```python
from build123d import *

# Parameters (mm, degrees)
F3_DEPTH = 1.3


with BuildPart() as f1:
    # F0 (on Front) → F1 (revolve)
    with BuildSketch(Plane.XZ):
        Polygon((-2.75, 0), (-1.5, 0), (-1.5, -10), (0, -10), (0, 0), (0, 3), (-2.75, 3), align=None)
    revolve(axis=Axis((0, 0, -5), (0, 0, 1)))

    # F2 (on face) → F3 (cut)
    with BuildSketch(Plane.XY.offset(3)):
        Polygon((-1.25, 0.721688), (-1.25, -0.721688), (0, -1.443376), (1.25, -0.721688), (1.25, 0.721688), (0, 1.443376), align=None)
    extrude(amount=-F3_DEPTH, mode=Mode.SUBTRACT)


solid = f1.part
```
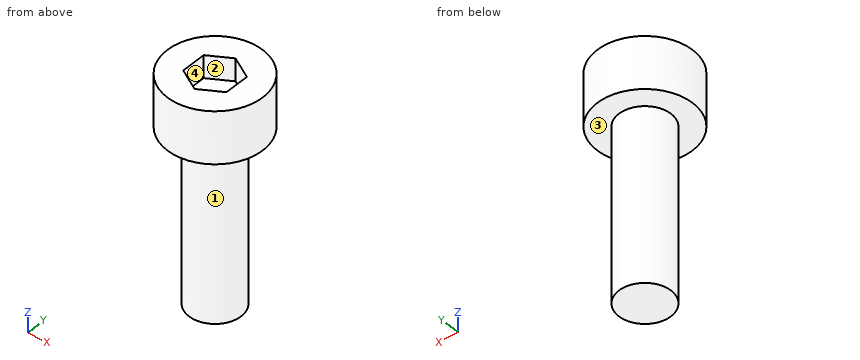
For this review, take the finished solid that the model builds, in its own axes (mm). Face numbers are marked on the shaded views. Give positions to 0.01 mm unless a question says otherwise; leave off trailing zeros. Write each loop counter-clockwise with the first axis right and the second up, starting at its lowest first coordinate (ties: lowest second). Pieces come first, ordered by that corner, then holes.
Item 1: Insertion check: P1, Ø0.6, axis at y = 0.5, z = 2, coming from the +X side; P2, Ø1, axis at x = 0, y = 0.5, coming from the +Z side; P3, Ø1.5, axis at x = 1.5, y = -2, coming from the -Z side. Each pin has a flat end and moves straight along its axis. Give the tip position at first contact, or say it passes through.
Item 2: Wall thickness on probe 1 along Z at (x, y) = (1.95, 1.5); probe 2 along Z at (x, y) = (-1.15, 0.4); probe 3 along Y at (x, z) = (0.55, 2.75): over which ranges is each line inside the solid? List them lowest first.
Item 3: Take a section at A-A (y = 0). Give the boundary of the cut face in (x, z).
Item 4: The part is to be moulded in two halves that separate along Y. For the marked faces 1, 2, 3 and 4, say which applies: +Y half, -Y half, draft (parallel to the pull), parting line (faces both ways), or undercut.
Item 5: Take a section at C-C (z = 1.25). Give the boundary of the cut face in (x, y).
Item 6: Take a section at D-D (y = -2.1). Give the boundary of the cut face in (x, z).
Item 7: Take a section at B-B (x = -0.6). Give the boundary of the cut face in (y, z).
Established:
1. P1: stops at x = 2.74
1. P2: stops at z = 1.7
1. P3: stops at z = 0
2. probe 1: z = 0 to 3
2. probe 2: z = -10 to 1.7
2. probe 3: y = -2.69 to -1.13, 1.13 to 2.69
3. outline: (-2.75, 0) - (-1.5, 0) - (-1.5, -10) - (1.5, -10) - (1.5, 0) - (2.75, 0) - (2.75, 3) - (1.25, 3) - (1.25, 1.7) - (-1.25, 1.7) - (-1.25, 3) - (-2.75, 3) - close
4. face 1: parting line
4. face 2: undercut
4. face 3: draft
4. face 4: undercut
5. outline: circle Ø5.5 at (0, 0)
6. outline: (-1.78, 0) - (1.78, 0) - (1.78, 3) - (-1.78, 3) - close
7. outline: (-2.68, 0) - (-1.37, 0) - (-1.37, -10) - (1.37, -10) - (1.37, 0) - (2.68, 0) - (2.68, 3) - (1.1, 3) - (1.1, 1.7) - (-1.1, 1.7) - (-1.1, 3) - (-2.68, 3) - close
